For this review, take the finished solid that the model builds, in its own axes (mm). A direction names the side the tool comes from. Give positions to 0.01 mm unless a question says otherwise; leave off trailing zeros. Order: outer loops, then holes, each group sorted by start corner. A loop starts at its lowest first (then second) coordinate and runs counter-clockwise, first axis right, second up.
from build123d import *

# Parameters (mm, degrees)
SKETCH1_W                          = 210.6
SKETCH1_H                          = 45
BASE_FLANGE1_DEPTH                 = 2
SM_EDGE_FLANGE_1_STRIP_W           = 10
SM_EDGE_FLANGE_1_STRIP_H           = 2
SM_EDGE_FLANGE_1_STRIP_CUT_DEPTH   = 45
SM_EDGE_FLANGE_1_STRIP_2_W         = 10
SM_EDGE_FLANGE_1_STRIP_2_H         = 2
SM_EDGE_FLANGE_1_STRIP_CUT_2_DEPTH = 45
SM_EDGE_FLANGE_1_DEPTH             = 45
SM_EDGE_FLANGE_1_BEND_DEPTH        = 45
SM_START                           = -20
SM_EDGE_FLANGE_2_DEPTH             = 20
SM_START_2                         = -3
SM_EDGE_FLANGE_2_2_DEPTH           = 3
SM_EDGE_FLANGE_2_3_DEPTH           = 17
SKETCH18_R                         = 1.55
CUT_EXTRUDE4_DEPTH                 = 10
CUT_EXTRUDE5_DEPTH                 = 213.740710726
CUT_EXTRUDE5_DEPTH_BACK            = 213.740710726
SKETCH22_W                         = 3
SKETCH22_H                         = 2
SKETCH22_H_2                       = 11.6


# Read off the part's stored shape, not the designer's step: Ребро-кромка2
# Sheet-metal steps are written as plain solids
with BuildPart() as part:
    # Sketch1 → Base-Flange1 (new body)
    with BuildSketch(Plane(origin=(0, 0, 0), x_dir=(1, 0, 0), z_dir=(0, 1, 0))):
        Rectangle(SKETCH1_W, SKETCH1_H)
    extrude(amount=-BASE_FLANGE1_DEPTH)

    # Ребро-кромка1 strip (across the edge) → Ребро-кромка1 strip cut (cut)
    with BuildSketch(Plane(origin=(-105.3, -2, 22.5), x_dir=(1, 0, 0), z_dir=(0, 0, -1))):
        with Locations((-2, -1)):
            Rectangle(SM_EDGE_FLANGE_1_STRIP_W, SM_EDGE_FLANGE_1_STRIP_H)
    extrude(amount=SM_EDGE_FLANGE_1_STRIP_CUT_DEPTH, mode=Mode.SUBTRACT)

    # Ребро-кромка1 strip 2 (across the edge) → Ребро-кромка1 strip cut 2 (cut)
    with BuildSketch(Plane(origin=(105.3, -2, -22.5), x_dir=(-1, 0, 0), z_dir=(0, 0, 1))):
        with Locations((-2, -1)):
            Rectangle(SM_EDGE_FLANGE_1_STRIP_2_W, SM_EDGE_FLANGE_1_STRIP_2_H)
    extrude(amount=SM_EDGE_FLANGE_1_STRIP_CUT_2_DEPTH, mode=Mode.SUBTRACT)

    # Ребро-кромка1 section (across the edge) → Ребро-кромка1 (add)
    with BuildSketch(Plane(origin=(-105.3, -2, 22.5), x_dir=(1, 0, 0), z_dir=(0, 0, -1))):
        with BuildLine():
            Line((0, 1), (0, 18))
            Line((0, 18), (2, 18))
            Line((2, 18), (2, 1))
            ThreePointArc((2, 1), (2.292893219, 0.292893219), (3, 0))
            Line((3, 0), (3, -2))
            ThreePointArc((3, -2), (0.878679656, -1.121320344), (0, 1))
        make_face()
    extrude(amount=SM_EDGE_FLANGE_1_DEPTH)

    # Ребро-кромка1 section 2 (across the edge) → Ребро-кромка1 bend (add)
    with BuildSketch(Plane(origin=(105.3, -2, -22.5), x_dir=(-1, 0, 0), z_dir=(0, 0, 1))):
        with BuildLine():
            Line((0, 1), (0, 18))
            Line((0, 18), (2, 18))
            Line((2, 18), (2, 1))
            ThreePointArc((2, 1), (2.292893219, 0.292893219), (3, 0))
            Line((3, 0), (3, -2))
            ThreePointArc((3, -2), (0.878679656, -1.121320344), (0, 1))
        make_face()
    extrude(amount=SM_EDGE_FLANGE_1_BEND_DEPTH)

    # Ребро-кромка2 outline → Ребро-кромка2 (cut)
    with BuildSketch(Plane(origin=(0, 0, 0), x_dir=(1, 0, 0), z_dir=(0, 1, 0)).offset(SM_START)):
        with BuildLine():
            Line((-102.3, -20.5), (-102.3, -19.5))
            Line((-102.3, -19.5), (-103.3, -19.5))
            ThreePointArc((-103.3, -19.5), (-103.007106781, -20.207106781), (-102.3, -20.5))
        make_face()
        with BuildLine():
            ThreePointArc((-102.3, -22.5), (-104.421320344, -21.621320344), (-105.3, -19.5))
            Line((-105.3, -19.5), (-105.3, -22.5))
            Line((-105.3, -22.5), (-102.3, -22.5))
        make_face()
        with BuildLine():
            Line((102.3, -22.5), (105.3, -22.5))
            Line((105.3, -22.5), (105.3, -19.5))
            ThreePointArc((105.3, -19.5), (104.421320344, -21.621320344), (102.3, -22.5))
        make_face()
        with BuildLine():
            Line((102.3, -19.5), (102.3, -20.5))
            ThreePointArc((102.3, -20.5), (103.007106781, -20.207106781), (103.3, -19.5))
            Line((103.3, -19.5), (102.3, -19.5))
        make_face()
    extrude(amount=SM_EDGE_FLANGE_2_DEPTH, mode=Mode.SUBTRACT)

    # Sm Edge Flange 2 2 outline → Sm Edge Flange 2 2 (cut)
    with BuildSketch(Plane(origin=(0, 0, 0), x_dir=(1, 0, 0), z_dir=(0, 1, 0)).offset(SM_START_2)):
        with BuildLine():
            Line((-102.3, -22.5), (-102.3, -20.5))
            ThreePointArc((-102.3, -20.5), (-103.007106781, -20.207106781), (-103.3, -19.5))
            Line((-103.3, -19.5), (-105.3, -19.5))
            ThreePointArc((-105.3, -19.5), (-104.421320344, -21.621320344), (-102.3, -22.5))
        make_face()
        with BuildLine():
            Line((102.3, -20.5), (102.3, -22.5))
            ThreePointArc((102.3, -22.5), (104.421320344, -21.621320344), (105.3, -19.5))
            Line((105.3, -19.5), (103.3, -19.5))
            ThreePointArc((103.3, -19.5), (103.007106781, -20.207106781), (102.3, -20.5))
        make_face()
    extrude(amount=SM_EDGE_FLANGE_2_2_DEPTH, mode=Mode.SUBTRACT)

    # Sm Edge Flange 2 3 outline → Sm Edge Flange 2 3 (add)
    with BuildSketch(Plane(origin=(0, 0, 0), x_dir=(1, 0, 0), z_dir=(0, 1, 0)).offset(SM_START)):
        with BuildLine():
            Line((93.3, -20.5), (93.3, -22.5))
            Line((93.3, -22.5), (102.3, -22.5))
            ThreePointArc((102.3, -22.5), (102.807305936, -22.456795679), (103.3, -22.328427125))
            Line((103.3, -22.328427125), (103.3, -19.5))
            ThreePointArc((103.3, -19.5), (103.007106781, -20.207106781), (102.3, -20.5))
            Line((102.3, -20.5), (93.3, -20.5))
        make_face()
        with BuildLine():
            Line((-93.3, -20.5), (-102.3, -20.5))
            ThreePointArc((-102.3, -20.5), (-103.007106781, -20.207106781), (-103.3, -19.5))
            Line((-103.3, -19.5), (-103.3, -22.328427125))
            ThreePointArc((-103.3, -22.328427125), (-102.807305936, -22.456795679), (-102.3, -22.5))
            Line((-102.3, -22.5), (-93.3, -22.5))
            Line((-93.3, -22.5), (-93.3, -20.5))
        make_face()
    extrude(amount=SM_EDGE_FLANGE_2_3_DEPTH)

    # Sketch18 → Cut-Extrude4 (cut)
    with BuildSketch(Plane(origin=(0, 0, 20.5), x_dir=(-1, 0, 0), z_dir=(0, 0, -1))):
        with Locations((-98.3, -17.3)):
            Circle(SKETCH18_R)
        with Locations((98.3, -17.3)):
            Circle(SKETCH18_R)
        with BuildLine():
            Line((-93.3, -2), (-102.3, -2))
            Line((-102.3, -2), (-102.3, -14.6))
            Line((-102.3, -14.6), (-98.3, -14.6))
            ThreePointArc((-98.3, -14.6), (-95.6, -17.3), (-98.3, -20))
            Line((-98.3, -20), (-93.3, -20))
            Line((-93.3, -20), (-93.3, -14.6))
            Line((-93.3, -14.6), (-93.3, -2))
        make_face()
        with BuildLine():
            Line((93.3, -14.6), (93.3, -20))
            Line((93.3, -20), (98.3, -20))
            ThreePointArc((98.3, -20), (95.6, -17.3), (98.3, -14.6))
            Line((98.3, -14.6), (102.3, -14.6))
            Line((102.3, -14.6), (102.3, -2))
            Line((102.3, -2), (93.3, -2))
            Line((93.3, -2), (93.3, -14.6))
        make_face()
    extrude(amount=-CUT_EXTRUDE4_DEPTH, mode=Mode.SUBTRACT)

    # Sketch22 → Cut-Extrude5 (cut, two sides: drawn at the far end of the back side and taken through both)
    with BuildSketch(Plane.ZY.offset(105.3).offset(-CUT_EXTRUDE5_DEPTH_BACK)):
        with Locations((21, -1)):
            Rectangle(SKETCH22_W, SKETCH22_H)
        Polygon((-22.5, -3), (19.5, -20), (-22.5, -20), align=None)
        with Locations((21, -8.8)):
            Rectangle(SKETCH22_W, SKETCH22_H_2)
    extrude(amount=CUT_EXTRUDE5_DEPTH + CUT_EXTRUDE5_DEPTH_BACK, mode=Mode.SUBTRACT)


solid = part.part
1) We need section C-C on z = 17. Give the boundary of the cut face in (x, y).
Answer sheet:
outline: (-105.3, -18.99) - (-103.3, -18.99) - (-103.3, -3) arc R1 cw to (-102.3, -2) - (102.3, -2) arc R1 cw to (103.3, -3) - (103.3, -18.99) - (105.3, -18.99) - (105.3, -3) arc R3 ccw to (102.3, 0) - (-102.3, 0) arc R3 ccw to (-105.3, -3) - close
2) To check wall thickness, follow line 1 (X direction, y = -6, z = -12); line 2 (Y direction, x = -98.3, z = 21.3); line 3 (Z direction, x = 70, y = -1). State the ranges of each line that lie inside material, in increasing order.
Answer sheet:
line 1: x = -105.3 to -103.3, 103.3 to 105.3
line 2: y = -20 to -18.85, -15.75 to -14.6
line 3: z = -22.5 to 19.5
3) We need section B-B on x = -51. Give the boundary of the cut face in (y, z), then the cut area to 3 significant figures.
Answer sheet:
outline: (-2, -22.5) - (0, -22.5) - (0, 19.5) - (-2, 19.5) - close
area: 84.0 mm2
4) Clearance check with flat-ended pins moving along their axes: pin 1 (4 mm diameter, centred on x = 98.3, y = -17.3, fed in from -Z); pin 2 (5 mm diameter, centred on x = -52.5, z = -2.5, fed in from -Y); pin 3 (0.9 mm diameter, centred on x = 102, z = 21, fed in from +Y). State where each tip first meets the part, or that it passes through.
Answer sheet:
pin 1: stops at z = 20.5
pin 2: stops at y = -2
pin 3: stops at y = -14.6
5) We need section A-A on z = -1.5. Give the boundary of the cut face in (x, y), then the cut area to 3 significant figures.
Answer sheet:
outline: (-105.3, -11.5) - (-103.3, -11.5) - (-103.3, -3) arc R1 cw to (-102.3, -2) - (102.3, -2) arc R1 cw to (103.3, -3) - (103.3, -11.5) - (105.3, -11.5) - (105.3, -3) arc R3 ccw to (102.3, 0) - (-102.3, 0) arc R3 ccw to (-105.3, -3) - close
area: 456 mm2
6) Draft analysis for pull direction X (two halves, no side actions). For faces 1 (the face through (104.314, -11.381, -1.794)), 2 (the face through (-1, -2, -2)), 3 (the face through (-103.3, -8, 8)), 4 (the face through (-105.3, -9, 3)), state which applies: +X half, -X half, draft (parallel to the pull), parting line (faces both ways), or undercut.
Answer sheet:
face 1: draft
face 2: undercut
face 3: undercut
face 4: -X half
7) Tool access review of faces 5 (the face through (100, -18, 20.5)), 6 (the face through (-104.286, -11.381, -1.794)): name each direction out of +Z, -Z, +X, -X, +Y, -Y from which nothing blocks a thin tool from reaching the whole face with its end or side.
Answer sheet:
face 5: -Z, +Y, -Y
face 6: -Z, +X, -X, -Y
